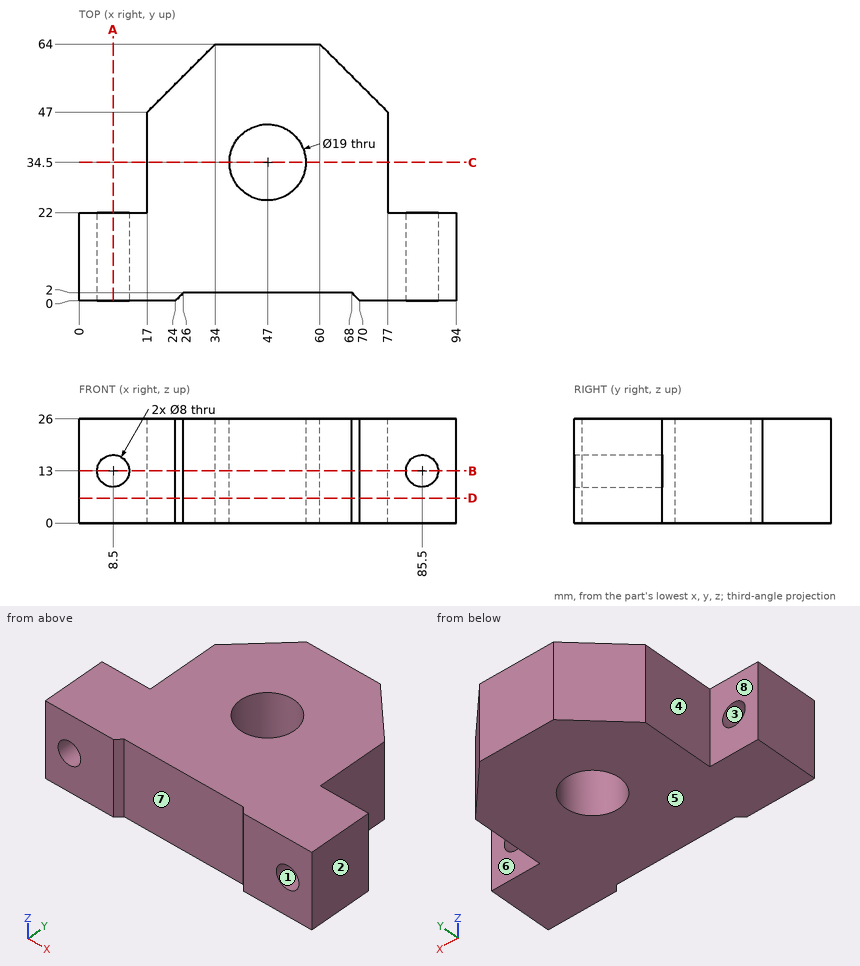
Here's the drawing with two shaded views (mm, measured from the low corner). I have some questions. A direction names the side the tool comes from. Give positions to 0.01 mm unless a question says otherwise; leave off trailing zeros. Write each loop counter-clockwise with the first axis right and the second up, starting at its lowest first coordinate (ties: lowest second). Pieces come first, ordered by that corner, then holes. Notation, with made-up numbers: (-12.75, 67) -> (7.25, 67) arc R20 ccw to (7.25, 97) -> close; hole circle Ø5 at (46, 42.5). An arc over 180 degrees is marked (long way). Use one line per item in the form item = value.
1) Suppose I cut it at D-D (z = 6.25). Please give me the cut outline in (x, y), and give its area (3 significant figures).
Verdict:
outline = (0, 0) -> (24, 0) -> (26, 2) -> (68, 2) -> (70, 0) -> (94, 0) -> (94, 22) -> (77, 22) -> (77, 47) -> (60, 64) -> (34, 64) -> (17, 47) -> (17, 22) -> (0, 22) -> close; hole circle Ø19 at (47, 34.5)
area = 3,930 mm2
2) We'd pull the mould along X, two halves only. Please class the marked faces 1, 2, 3 and 4: +X half, -X half, draft (parallel to the pull), parting line (faces both ways), or undercut.
Verdict:
face_1 = undercut
face_2 = +X half
face_3 = undercut
face_4 = -X half
3) On a 3-axis mill with a long thin cutter (end or side, diameter ignored), from which of +Z, -Z, +X, -X, +Y, -Y can I reach the whole of each face in a straight line? I mean the marked faces 5, 6, 7 and 8. Say none if no direction works.
Verdict:
face_5 = -Z, +X, -X, +Y, -Y
face_6 = +Z, -Z, +X, +Y
face_7 = +Z, -Z, -Y
face_8 = +Z, -Z, -X, +Y
4) Suppose I cut it at C-C (y = 34.5). Please give me the cut outline in (x, z).
Verdict:
outline = (17, 0) -> (37.5, 0) -> (37.5, 26) -> (17, 26) -> close; (56.5, 0) -> (77, 0) -> (77, 26) -> (56.5, 26) -> close
5) Suppose I cut it at B-B (z = 13). Please give me the cut outline in (x, y), and give its area (3 significant figures).
Verdict:
outline = (0, 0) -> (4.5, 0) -> (4.5, 22) -> (0, 22) -> close; (12.5, 0) -> (24, 0) -> (26, 2) -> (68, 2) -> (70, 0) -> (81.5, 0) -> (81.5, 22) -> (77, 22) -> (77, 47) -> (60, 64) -> (34, 64) -> (17, 47) -> (17, 22) -> (12.5, 22) -> close; (89.5, 0) -> (94, 0) -> (94, 22) -> (89.5, 22) -> close; hole circle Ø19 at (47, 34.5)
area = 3,580 mm2
6) If I drill on L1, parallel to Z at x = 85.5, y = 14; L2, parallel to X at y = 15.75, z = 13; L3, parallel to Y at x = 47, z = 20.5, over which ranges is the centre line in solid material (lowest first)? Write a range as [from, to].
Verdict:
L1 = [0, 9], [17, 26]
L2 = [0, 4.5], [12.5, 81.5], [89.5, 94]
L3 = [2, 25], [44, 64]
7) I'm going to push flat-ended pins straight in: pin 1 (5 mm diameter, centred on y = 43.5, z = 15.5, fed in from +X); pin 2 (8 mm diameter, centred on x = 43, z = 14, fed in from -Y); pin 3 (8.5 mm diameter, centred on x = 88, z = 8.5, fed in from +Y); pin 4 (13 mm diameter, centred on x = 85.5, z = 13, fed in from -Y). Where does each tip first touch, or does it pass through?
Verdict:
pin_1 = 77
pin_2 = 2
pin_3 = 22
pin_4 = 0
8) Suppose I cut it at A-A (x = 8.5). Please give me the cut outline in (y, z), and give its area (3 significant figures).
Verdict:
outline = (0, 0) -> (22, 0) -> (22, 9) -> (0, 9) -> close; (0, 17) -> (22, 17) -> (22, 26) -> (0, 26) -> close
area = 396 mm2
